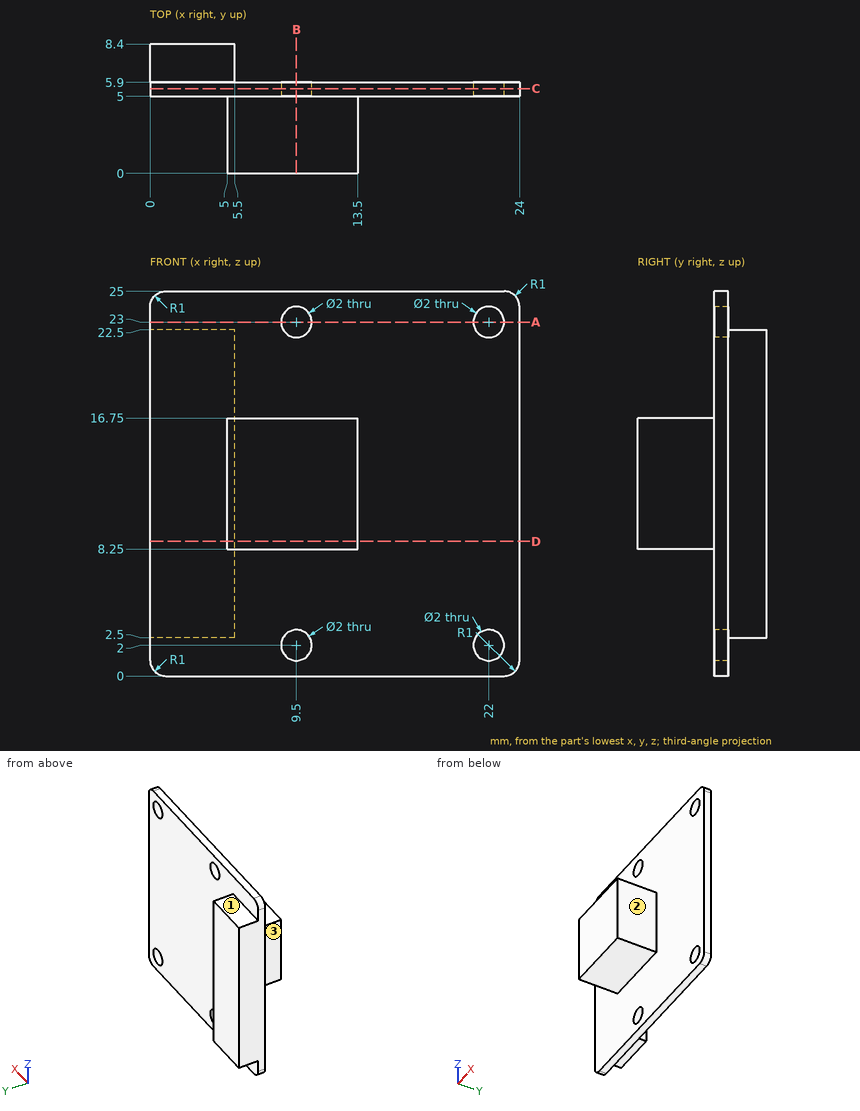
Design review of the part shown in the three views and the two pictorial views. Dimensions are in mm from the part's minimum x, y and z. A direction names the side the tool comes from. Give positions to 0.01 mm unless a question says otherwise; leave off trailing zeros. Loops run counter-clockwise (first coordinate to the right, second up) from the corner with the lowest first, then second, coordinate; pieces in that order, holes last. Notation, with made-up numbers: (3, -40) -> (34, -40) arc R19 ccw to (34, -20) -> close; hole circle Ø2 at (15.5, 10). An arc over 180 degrees is marked (long way). Answer as a JSON object with one key per item and string values. Group by question number.
Q1. Wall thickness on line 1 along Z through (x, y) = (22, 5.45); line 2 along Y through (x, z) = (11.75, 1); line 3 along Y through (x, z) = (12.75, 15.5): over which ranges is each line inside the solid? List them lowest first.
Q2. Take a section at A-A (z = 23). Write out the cut boundary in (x, y), plus the area to 3 significant figures.
Q3. Take a section at D-D (z = 8.75). Write out the cut boundary in (x, y).
Q4. Tool access review of the marked faces 1, 2 and 3: name each direction out of +Z, -Z, +X, -X, +Y, -Y from which nothing blocks a thin tool from reaching the whole face with its end or side.
Q5. Take a section at C-C (y = 5.5). Write out the cut boundary in (x, z), plus the area to 3 significant figures.
Q6. Take a section at B-B (x = 9.5). Write out the cut boundary in (y, z), plus the area to 3 significant figures.
Q7. Insertion check: pin 1 (2 mm diameter, centred on x = 3.5, z = 9, fed in from -Y); pin 2 (2 mm diameter, centred on y = 3.5, z = 10, fed in from -X); pin 3 (4 mm diameter, centred on x = 10, y = 2, fed in from -Z). Each pin has a flat end and moves straight along its axis. Give the tip position at first contact, or say it passes through.
Answer below:
{
 "1": {"line 1": "z = 0 to 1, 3 to 22, 24 to 25", "line 2": "y = 5 to 5.9", "line 3": "y = 0 to 5.9"},
 "2": {"outline": "(0, 5) -> (8.5, 5) -> (8.5, 5.9) -> (0, 5.9) -> close; (10.5, 5) -> (21, 5) -> (21, 5.9) -> (10.5, 5.9) -> close; (23, 5) -> (24, 5) -> (24, 5.9) -> (23, 5.9) -> close", "area": "18.0 mm2"},
 "3": {"outline": "(0, 5) -> (5, 5) -> (5, 0) -> (13.5, 0) -> (13.5, 5) -> (24, 5) -> (24, 5.9) -> (5.5, 5.9) -> (5.5, 8.4) -> (0, 8.4) -> close"},
 "4": {"face 1": "+Z, +X, -X, +Y", "face 2": "+Z, -Z, +X, -Y", "face 3": "+Z, -Z, -X, -Y"},
 "5": {"outline": "(0, 1) arc R1 ccw to (1, 0) -> (23, 0) arc R1 ccw to (24, 1) -> (24, 24) arc R1 ccw to (23, 25) -> (1, 25) arc R1 ccw to (0, 24) -> close; hole circle Ø2 at (9.5, 2); hole circle Ø2 at (9.5, 23); hole circle Ø2 at (22, 2); hole circle Ø2 at (22, 23)", "area": "587 mm2"},
 "6": {"outline": "(0, 8.25) -> (5, 8.25) -> (5, 3) -> (5.9, 3) -> (5.9, 22) -> (5, 22) -> (5, 16.75) -> (0, 16.75) -> close; (5, 0) -> (5.9, 0) -> (5.9, 1) -> (5, 1) -> close; (5, 24) -> (5.9, 24) -> (5.9, 25) -> (5, 25) -> close", "area": "61.4 mm2"},
 "7": {"pin 1": "stops at y = 5", "pin 2": "stops at x = 5", "pin 3": "stops at z = 8.25"}
}
